For this review, take the finished solid that the model builds, in its own axes (mm). Round coordinates to 2 decimals unless told otherwise and drop trailing zeros. Loops run counter-clockwise (first coordinate to the right, second up) from the corner with the lowest first, then second, coordinate; pieces in that order, holes last.
1. To check wall thickness, follow line 1 along Z through (x, y) = (4.5, 0.2); line 2 along X through (y, z) = (2.6, -34.5); line 3 along X through (y, z) = (0.75, -30.5). State the ranges of each line that lie inside material, in increasing order.
2. Consider section A-A on z = -32. State the section outline as (x, y) points, then the cut area to 3 significant figures.
3. Consider section C-C on y = 1.7. State the section outline as (x, z) points.
4. Consider section B-B on x = -9.5. State the section outline as (y, z) points, then the cut area to 3 significant figures.
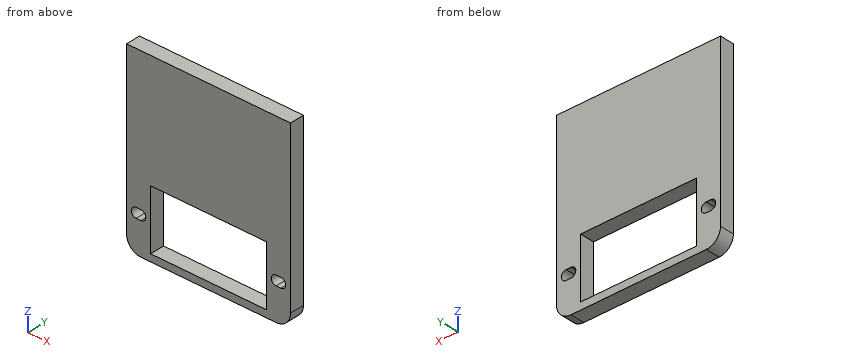
from build123d import *

# Parameters (mm, degrees)
BOSS_EXTRU_1_DEPTH = 3
CONG_1_R           = 3
CONG_2_R           = 3


with BuildPart() as part:
    # Esquisse1 → Boss.-Extru.1 (new body)
    with BuildSketch(Plane(origin=(0, 0, 0), x_dir=(1, 0, 0), z_dir=(0, 1, 0))):
        Polygon((-12.05, 36.5), (0, 36.5), (0, 38), (-17.05, 38), (-17.05, 0), (0, 0), (0, 24), (-12.05, 24), align=None)
        with BuildLine():
            ThreePointArc((-15.05, 29.25), (-16.05, 30.25), (-15.05, 31.25))
            Line((-15.05, 31.25), (-14.05, 31.25))
            ThreePointArc((-14.05, 31.25), (-13.05, 30.25), (-14.05, 29.25))
            Line((-14.05, 29.25), (-15.05, 29.25))
        make_face(mode=Mode.SUBTRACT)
    boss_extru_1 = extrude(amount=BOSS_EXTRU_1_DEPTH)

    # Symétrie1: Boss.-Extru.1 across plane
    add(boss_extru_1.mirror(Plane(origin=(0, 3, 0), x_dir=(0, 0, 1), z_dir=(-1, 0, 0))))

    # Congé1
    cong_1_edges = [part.edges().sort_by_distance(p)[0] for p in [
        (17.05, 1.5, -38),
    ]]
    fillet(cong_1_edges, radius=CONG_1_R)

    # Congé2
    cong_2_edges = [part.edges().sort_by_distance(p)[0] for p in [
        (-17.05, 1.5, -38),
    ]]
    fillet(cong_2_edges, radius=CONG_2_R)


solid = part.part
Resolved:
1. line 1: z = -38 to -36.5, -24 to 0
1. line 2: x = -17.05 to -12.05, 12.05 to 17.05
1. line 3: x = -17.05 to -16.02, -13.08 to -12.05, 12.05 to 13.08, 16.02 to 17.05
2. outline: (-17.05, 0) - (-12.05, 0) - (-12.05, 3) - (-17.05, 3) - close; (12.05, 0) - (17.05, 0) - (17.05, 3) - (12.05, 3) - close
2. area: 30.0 mm2
3. outline: (-17.05, -35) arc R3 ccw to (-14.05, -38) - (14.05, -38) arc R3 ccw to (17.05, -35) - (17.05, 0) - (-17.05, 0) - close; hole (-15.05, -31.25) - (-14.05, -31.25) arc R1 ccw to (-14.05, -29.25) - (-15.05, -29.25) arc R1 ccw to start; hole (-12.05, -36.5) - (12.05, -36.5) - (12.05, -24) - (-12.05, -24) - close; hole (14.05, -31.25) - (15.05, -31.25) arc R1 ccw to (15.05, -29.25) - (14.05, -29.25) arc R1 ccw to start
4. outline: (0, -38) - (3, -38) - (3, -36.5) - (0, -36.5) - close; (0, -24) - (3, -24) - (3, 0) - (0, 0) - close
4. area: 76.5 mm2
